Read the model definition and answer for the solid it produces. Units are mm, in the model's axes. A direction names the side the tool comes from. Give positions to 0.01 mm unless a question says otherwise; leave off trailing zeros. Loops run counter-clockwise (first coordinate to the right, second up) from the corner with the lowest first, then second, coordinate; pieces in that order, holes last. Notation, with made-up numbers: (17.25, 17) -> (76.25, 17) arc R23 ccw to (76.25, 26) -> close; hole circle Ø2 at (60.25, -28). An arc over 180 degrees is marked (long way). Write each question's results on one line, items separated by ' | '. Start each with the question number.
Item 1: Which of the six approach directions +Z, -Z, +X, -X, +Y, -Y give full straight-line access (tool end or side, diameter ignored) to faces 4 (the cylindrical face through (3.688, -1.548, -3.451)), 5 (the cylindrical face through (-3, 0, -3)), 6 (the flat face through (-17, -0.25, -4))?
Item 2: Section D-D on x = 5.5 is taken. Write down the section's boundary in (y, z), and give its area (3 significant figures).
Item 3: Section C-C on x = -15 is taken. Write down the section's boundary in (y, z).
Item 4: Determine the mould class of faces 1 (the flat face through (0, 0, 0)), 2 (the flat face through (-20.175, -20.17, -3.451)), 3 (the flat face through (-28.5, 0, -3.5)) for opening direction Y: +Y half, -Y half, draft (parallel to the pull), parting line (faces both ways), or undercut.
Item 5: Find the intervals of material crossed by line 1 (X direction, y = -13.5, z = -4.75); line 2 (X direction, y = 18.5, z = -1.5); line 3 (Y direction, x = -24, z = -2.75), in increasing order.
Item 6: Section A-A on y = 9 is taken. Write down the section's boundary in (x, z), and give its area (3 significant figures).
Item 7: Each of these flat-tipped pins is pushed along its axis until it touches: P1, Ø5, axis at x = 23.5, y = -22, coming from the +Z side; P2, Ø4, axis at y = -13, z = -1.5, coming from the -X side; P3, Ø3.5, axis at x = -3.5, y = -7.5, coming from the -Z side; P4, Ø1.5, axis at x = 16.5, y = -13, coming from the -Z side. Where does it stop, or does it pass through?
```python
from build123d import *

# Parameters (mm, degrees)
BOSS_EXTRUDE1_DEPTH = 5
SKETCH2_R           = 10
BOSS_EXTRUDE2_DEPTH = 2
SKETCH4_R           = 4
SKETCH4_R_2         = 3
BOSS_EXTRUDE3_DEPTH = 7
BOSS_EXTRUDE5_DEPTH = 0.25
CIRPATTERN1_COUNT   = 8
BOSS_EXTRUDE6_DEPTH = 2


with BuildPart() as part:
    # Sketch1 → Boss-Extrude1 (new body)
    with BuildSketch(Plane.XY):
        Polygon((-0.738715324, 1.305488288), (-1.499943684, 0.012997907), (-0.76122836, -1.292490381), (0.738715324, -1.305488288), (1.499943684, -0.012997907), (0.76122836, 1.292490381), align=None)
    extrude(amount=BOSS_EXTRUDE1_DEPTH)

    # Sketch2 → Boss-Extrude2 (add)
    with BuildSketch(Plane.XY):
        Circle(SKETCH2_R)
    extrude(amount=BOSS_EXTRUDE2_DEPTH)

    # Sketch4 → Boss-Extrude3 (add)
    with BuildSketch(Plane.XY):
        Circle(SKETCH4_R)
        Circle(SKETCH4_R_2, mode=Mode.SUBTRACT)
    extrude(amount=-BOSS_EXTRUDE3_DEPTH)

    # Sketch7 → Boss-Extrude5 (add, symmetric)
    with BuildSketch(Plane(origin=(0, 0, 0), x_dir=(0, 0, -1), z_dir=(1, 0, 0))):
        Polygon((7, 3.5), (0, 3.5), (0, 30.5), (7, 26.5), align=None)
    boss_extrude5 = extrude(amount=BOSS_EXTRUDE5_DEPTH, both=True)

    # CirPattern1: Boss-Extrude5 ×8 about axis
    cirpattern1_axis = Axis((0, 0, 0), (0, 0, 1))
    for i in range(1, CIRPATTERN1_COUNT):
        add(boss_extrude5.rotate(cirpattern1_axis, i * 360 / CIRPATTERN1_COUNT))

    # Sketch9 → Boss-Extrude6 (add)
    with BuildSketch(Plane(origin=(-1.499943684, 0.012997907, 5), x_dir=(-1, 0, 0), z_dir=(0, 0, -1))):
        Polygon((-0.76122836, 1.292490381), (-2.261172044, 1.279492473), (-2.999887367, -0.025995815), (-2.238659008, -1.318486195), (-0.738715324, -1.305488288), (0, 0), align=None)
    extrude(amount=-BOSS_EXTRUDE6_DEPTH)


solid = part.part
```
Findings:
1) face 4: -Z, +X | face 5: -Z | face 6: -Z, -X
2) outline: (-8.35, 0) -> (-5.85, 0) -> (-5.85, -7) -> (-5.15, -7) -> (-5.15, 0) -> (-0.25, 0) -> (-0.25, -7) -> (0.25, -7) -> (0.25, 0) -> (5.15, 0) -> (5.15, -7) -> (5.85, -7) -> (5.85, 0) -> (8.35, 0) -> (8.35, 2) -> (-8.35, 2) -> close | area: 46.8 mm2
3) outline: (-15.35, -7) -> (-14.65, -7) -> (-14.65, 0) -> (-15.35, 0) -> close; (-0.25, -7) -> (0.25, -7) -> (0.25, 0) -> (-0.25, 0) -> close; (14.65, -7) -> (15.35, -7) -> (15.35, 0) -> (14.65, 0) -> close
4) face 1: undercut | face 2: -Y half | face 3: draft
5) line 1: -13.85 to -13.15, -0.25 to 0.25, 13.15 to 13.85 | line 2: -18.85 to -18.15, -0.25 to 0.25, 18.15 to 18.85 | line 3: -0.25 to 0.25
6) outline: (-9.35, -7) -> (-8.65, -7) -> (-8.65, 0) -> (-9.35, 0) -> close; (-4.36, 0) -> (-0.25, 0) -> (-0.25, -7) -> (0.25, -7) -> (0.25, 0) -> (4.36, 0) -> (4.36, 2) -> (-4.36, 2) -> close; (8.65, -7) -> (9.35, -7) -> (9.35, 0) -> (8.65, 0) -> close | area: 30.8 mm2
7) P1: z = 0 | P2: x = -15.35 | P3: z = 0 | P4: through
